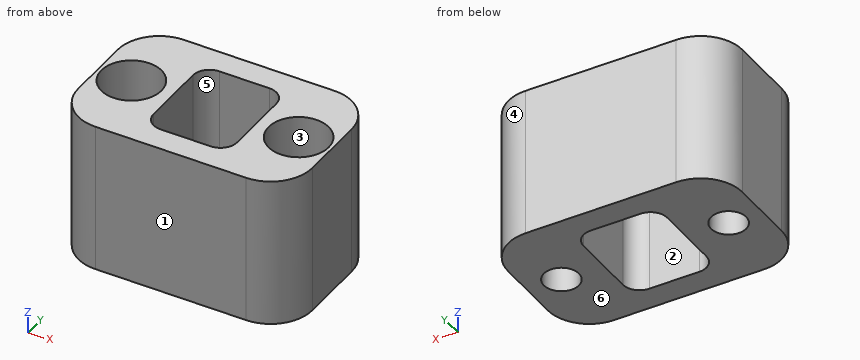
```python
from build123d import *

# Parameters (mm, degrees)
SKETCH_1_W          = 28
SKETCH_1_H          = 18
SKETCH_1_R          = 2.1
EXTRUDE_1_DEPTH     = 18
SKETCH_2_R          = 3.6
CUT_EXTRUDE_1_DEPTH = 15
SKETCH_3_W          = 10
SKETCH_3_H          = 12
CUT_EXTRUDE_2_DEPTH = 25
FILLET_1_R          = 2
FILLET_2_R          = 5


with BuildPart() as part:
    # 草图1 → 凸台-拉伸1 (new body)
    with BuildSketch(Plane.XY):
        Rectangle(SKETCH_1_W, SKETCH_1_H)
        with Locations((-10, 0)):
            Circle(SKETCH_1_R, mode=Mode.SUBTRACT)
        with Locations((10, 0)):
            Circle(SKETCH_1_R, mode=Mode.SUBTRACT)
    extrude(amount=EXTRUDE_1_DEPTH)

    # 草图2 → 切除-拉伸1 (cut)
    with BuildSketch(Plane.XY.offset(18)):
        with Locations((-10, 0)):
            Circle(SKETCH_2_R)
        with Locations((10, 0)):
            Circle(SKETCH_2_R)
    extrude(amount=-CUT_EXTRUDE_1_DEPTH, mode=Mode.SUBTRACT)

    # 草图3 → 切除-拉伸2 (cut)
    with BuildSketch(Plane.XY.offset(18)):
        Rectangle(SKETCH_3_W, SKETCH_3_H)
    extrude(amount=-CUT_EXTRUDE_2_DEPTH, mode=Mode.SUBTRACT)

    # 圆角1
    fillet_1_edges = [part.edges().sort_by_distance(p)[0] for p in [
        (5, 6, 9),
        (5, -6, 9),
        (-5, -6, 9),
        (-5, 6, 9),
    ]]
    fillet(fillet_1_edges, radius=FILLET_1_R)

    # 圆角2
    fillet_2_edges = [part.edges().sort_by_distance(p)[0] for p in [
        (14, -9, 9),
        (-14, -9, 9),
        (-14, 9, 9),
        (14, 9, 9),
    ]]
    fillet(fillet_2_edges, radius=FILLET_2_R)


solid = part.part
```
CAD build for the part. Positions are in the model's coordinates, mm. Face numbers are marked on the shaded views. A direction names the side the tool comes from. Give positions to 0.01 mm unless a question says otherwise; leave off trailing zeros. Order: outer loops, then holes, each group sorted by start corner. A loop starts at its lowest first (then second) coordinate and runs counter-clockwise, first axis right, second up.
(1) Saw through at A-A, the plane z = 4.75. Give the cut face in (x, y).
(2) Flat gauge pins, fed straight in: pin 1 (4.5 mm diameter, centred on x = -10, y = 0, fed in from +Z); pin 2 (1 mm diameter, centred on x = 10, z = 14.5, fed in from -Y). Where does each tip first touch, or does it go through?
(3) Mould opens along Y. For the marked faces 4, 5 and 6 say: released by +Y, released by -Y, zero draft, split by the parting line, or undercut.
(4) Saw through at B-B, the plane y = 0. Give the cut face in (x, z), then the cut area to 3 significant figures.
(5) Drill centre lines: L1, parallel to X at y = 0, z = 2.15; L2, parallel to X at y = 0.5, z = 16; L3, parallel to Y at x = -2.25, z = 16. Where is each one in solid material? Low to high.
(6) Saw through at D-D, the plane y = -2.75. Give the cut face in (x, z), then the cut area to 3 significant figures.
(7) Saw through at C-C, the plane x = 11.5. Give the cut face in (y, z).
(8) Tool access for the marked faces 1, 2 and 3: list every direction of +Z, -Z, +X, -X, +Y, -Y with a clear straight run to the whole face (end or side of a thin tool).
Results found:
1. outline: (-14, -4) arc R5 ccw to (-9, -9) - (9, -9) arc R5 ccw to (14, -4) - (14, 4) arc R5 ccw to (9, 9) - (-9, 9) arc R5 ccw to (-14, 4) - close; hole circle Ø7.2 at (-10, 0); hole (-5, -4) arc R2 ccw to (-3, -6) - (3, -6) arc R2 ccw to (5, -4) - (5, 4) arc R2 ccw to (3, 6) - (-3, 6) arc R2 ccw to (-5, 4) - close; hole circle Ø7.2 at (10, 0)
2. pin 1: stops at z = 3
2. pin 2: stops at y = -8.97
3. face 4: released by +Y
3. face 5: undercut
3. face 6: zero draft
4. outline: (-14, 0) - (-12.1, 0) - (-12.1, 3) - (-13.6, 3) - (-13.6, 18) - (-14, 18) - close; (-7.9, 0) - (-5, 0) - (-5, 18) - (-6.4, 18) - (-6.4, 3) - (-7.9, 3) - close; (5, 0) - (7.9, 0) - (7.9, 3) - (6.4, 3) - (6.4, 18) - (5, 18) - close; (12.1, 0) - (14, 0) - (14, 18) - (13.6, 18) - (13.6, 3) - (12.1, 3) - close
4. area: 82.8 mm2
5. L1: x = -14 to -12.1, -7.9 to -5, 5 to 7.9, 12.1 to 14
5. L2: x = -14 to -13.57, -6.43 to -5, 5 to 6.43, 13.57 to 14
5. L3: y = -9 to -6, 6 to 9
6. outline: (-14, 0) - (-5, 0) - (-5, 18) - (-7.68, 18) - (-7.68, 3) - (-12.32, 3) - (-12.32, 18) - (-14, 18) - close; (5, 0) - (14, 0) - (14, 18) - (12.32, 18) - (12.32, 3) - (7.68, 3) - (7.68, 18) - (5, 18) - close
6. area: 185 mm2
7. outline: (-8.33, 0) - (-1.47, 0) - (-1.47, 3) - (-3.27, 3) - (-3.27, 18) - (-8.33, 18) - close; (1.47, 0) - (8.33, 0) - (8.33, 18) - (3.27, 18) - (3.27, 3) - (1.47, 3) - close
8. face 1: +Z, -Z, +X, -X, -Y
8. face 2: +Z, -Z
8. face 3: +Z
